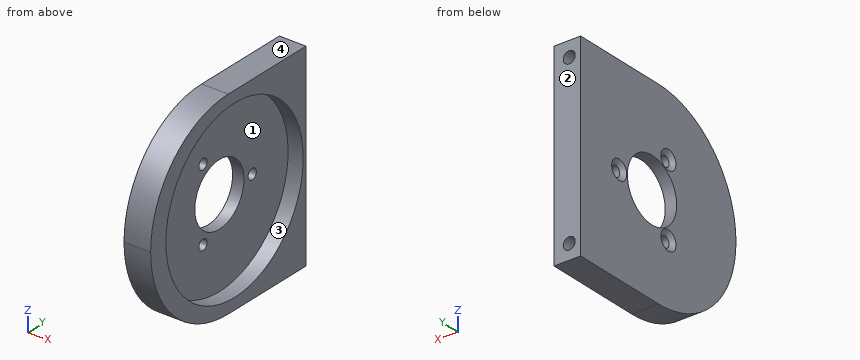
from build123d import *

# Parameters (mm, degrees)
ESBO_O1_W                                            = 52
ESBO_O1_H                                            = 52
RESSALTO_EXTRUS_O1_DEPTH                             = 7
ESBO_O2_R                                            = 8.25
CORTE_EXTRUS_O1_DEPTH                                = 74.87151007
ESCAREADO_PARA_PARAFUSO_DE_M_QUINA_COM_C_D           = 2.794
ESCAREADO_PARA_PARAFUSO_DE_M_QUINA_COM_C_CSINK_D     = 5.0546
ESCAREADO_PARA_PARAFUSO_DE_M_QUINA_COM_C_CSINK_ANGLE = 100
PADR_OCIRCULAR1_COUNT                                = 3
ESBO_O27_R                                           = 23
CORTE_EXTRUS_O5_DEPTH                                = 4
FILETE1_R                                            = 26
FURO_ROSCADO_PARA_CONDU_TE_DE_M3X0_51_D              = 3.15
FURO_ROSCADO_PARA_CONDU_TE_DE_M3X0_51_DEPTH          = 10
FURO_ROSCADO_PARA_CONDU_TE_DE_M3X0_51_TIP            = 0.946355475


with BuildPart() as part:
    # Esboço1 → Ressalto-extrusão1 (new body)
    with BuildSketch(Plane(origin=(0, 0, 0), x_dir=(0, 0, -1), z_dir=(1, 0, 0))):
        with Locations((26, 26)):
            Rectangle(ESBO_O1_W, ESBO_O1_H)
    extrude(amount=RESSALTO_EXTRUS_O1_DEPTH)

    # Esboço2 → Corte-extrusão1 (cut, through all)
    with BuildSketch(Plane.ZY):
        with Locations((-26, 28.1)):
            Circle(ESBO_O2_R)
    extrude(amount=-CORTE_EXTRUS_O1_DEPTH, mode=Mode.SUBTRACT)

    # Escareado para parafuso de máquina com cabeça chata (100) de #32 (through all)
    with Locations(Plane.ZY):
        with Locations((-26, 39.1)):
            escareado_para_parafuso_de_m_quina_com_c = CounterSinkHole(ESCAREADO_PARA_PARAFUSO_DE_M_QUINA_COM_C_D / 2, ESCAREADO_PARA_PARAFUSO_DE_M_QUINA_COM_C_CSINK_D / 2, counter_sink_angle=ESCAREADO_PARA_PARAFUSO_DE_M_QUINA_COM_C_CSINK_ANGLE)

    # PadrãoCircular1: Escareado para parafuso de máquina com cabeça chata (100) de #32 ×3 about axis
    padr_ocircular1_axis = Axis((0, 28.1, -26), (1, 0, 0))
    for i in range(1, PADR_OCIRCULAR1_COUNT):
        add(escareado_para_parafuso_de_m_quina_com_c.rotate(padr_ocircular1_axis, i * 360 / PADR_OCIRCULAR1_COUNT), mode=Mode.SUBTRACT)

    # Esboço27 → Corte-extrusão5 (cut)
    with BuildSketch(Plane(origin=(7, 0, 0), x_dir=(0, 0, -1), z_dir=(1, 0, 0))):
        with Locations((26, 28.1)):
            Circle(ESBO_O27_R)
    extrude(amount=-CORTE_EXTRUS_O5_DEPTH, mode=Mode.SUBTRACT)

    # Filete1
    filete1_edges = [part.edges().sort_by_distance(p)[0] for p in [
        (3.5, 0, -52),
        (3.5, 0, 0),
    ]]
    fillet(filete1_edges, radius=FILETE1_R - 0.0001)  # a hair under: the kernel refuses the full size

    # Furo roscado para conduíte de M3x0.51
    with Locations(Plane(origin=(0, 52, 0), x_dir=(1, 0, 0), z_dir=(0, 1, 0))):
        with Locations((3, 48), (3, 4)):
            Hole(FURO_ROSCADO_PARA_CONDU_TE_DE_M3X0_51_D / 2, depth=FURO_ROSCADO_PARA_CONDU_TE_DE_M3X0_51_DEPTH)
            with Locations((0, 0, -(FURO_ROSCADO_PARA_CONDU_TE_DE_M3X0_51_DEPTH + FURO_ROSCADO_PARA_CONDU_TE_DE_M3X0_51_TIP / 2))):  # 118° drill point
                Cone(0, FURO_ROSCADO_PARA_CONDU_TE_DE_M3X0_51_D / 2, FURO_ROSCADO_PARA_CONDU_TE_DE_M3X0_51_TIP, mode=Mode.SUBTRACT)


solid = part.part
For this review, take the finished solid that the model builds, in its own axes (mm). Face numbers are marked on the shaded views. Give positions to 0.01 mm unless a question says otherwise; leave off trailing zeros. Order: outer loops, then holes, each group sorted by start corner. A loop starts at its lowest first (then second) coordinate and runs counter-clockwise, first axis right, second up. Notation, with made-up numbers: (15, 44.25) - (21, 44.25) arc R7 cw to (21, 57.25) - close; hole circle Ø11 at (85, 50.25). An arc over 180 degrees is marked (long way). Answer as a JSON object with one key per item and string values. Group by question number.
Item 1: Draft analysis for pull direction Y (two halves, no side actions). For the marked faces 1, 2, 3 and 4, state which applies: pulls with the +Y half, pulls with the -Y half, needs draft (parallel to the pull), parting line crosses it, or undercut.
Item 2: Take a section at A-A on y = 28.1. Give the boundary of the cut face in (x, z).
Item 3: Take a section at D-D on z = -40.5. Give the boundary of the cut face in (x, y).
Item 4: Take a section at C-C on y = 22.6. Give the boundary of the cut face in (x, z).
Item 5: Clearance check with flat-ended pins moving along their axes: pin 1 Ø3 at (x, y) = (3, 24.5) entering from +Z; pin 2 Ø2 at (y, z) = (24.5, -37) entering from +X; pin 3 Ø2.5 at (x, z) = (3, -48) entering from -Y; pin 4 Ø3.5 at (x, z) = (3, -4) entering from -Y. State where each tip first meets the part, or that it passes through.
Item 6: Wall thickness on line 1 along Y through (x, z) = (4.55, -26); line 2 along Z through (x, y) = (2.2, 22.6); line 3 along Y through (x, z) = (2.15, -26): over which ranges is each line inside the solid? List them lowest first.
Reported:
{
 "1": {"face 1": "undercut", "face 2": "pulls with the +Y half", "face 3": "undercut", "face 4": "needs draft"},
 "2": {"outline": "(0, -52) - (7, -52) - (7, -49) - (3, -49) - (3, -34.25) - (0, -34.25) - close; (0, -17.75) - (3, -17.75) - (3, -3) - (7, -3) - (7, 0) - (0, 0) - close"},
 "3": {"outline": "(0, 4.42) - (7, 4.42) - (7, 10.25) - (3, 10.25) - (3, 45.95) - (7, 45.95) - (7, 52) - (0, 52) - close"},
 "4": {"outline": "(0, -51.78) - (7, -51.78) - (7, -48.33) - (3, -48.33) - (3, -36.92) - (0.95, -36.92) - (0, -38.05) - close; (0, -33) - (0.95, -34.13) - (3, -34.13) - (3, -32.15) - (0, -32.15) - close; (0, -19.85) - (3, -19.85) - (3, -17.87) - (0.95, -17.87) - (0, -19) - close; (0, -13.95) - (0.95, -15.08) - (3, -15.08) - (3, -3.67) - (7, -3.67) - (7, -0.22) - (0, -0.22) - close"},
 "5": {"pin 1": "z = 0", "pin 2": "x = 3", "pin 3": "y = 10.33", "pin 4": "y = 9.69"},
 "6": {"line 1": "0 to 5.1, 51.1 to 52", "line 2": "-51.78 to -36.92, -34.13 to -32.15, -19.85 to -17.87, -15.08 to -0.22", "line 3": "0 to 19.85, 36.35 to 37.7, 40.5 to 52"}
}
